Study the drawing (mm; zero at the part's minimum x, y, z) and answer. A direction names the side the tool comes from. Give positions to 0.01 mm unless a question says otherwise; leave off trailing zeros. Order: outer loops, then holes, each group sorted by start corner. A loop starts at its lowest first (then second) coordinate and runs counter-clockwise, first axis right, second up. Notation, with made-up numbers: (-1, -29.75) - (29, -29.75) arc R20 cw to (29, -18.75) - close; hole circle Ø4 at (-30.75, -38). An arc over 180 degrees is marked (long way). Write each question's results on one line, items separated by ' | '. Start each with the question number.
Q1. Find section A-A on z = 34.5. Count the separate pieces of the cut face and the enclosed holes in it, and give its area (3 significant figures).
Q2. Flat-ended cylindrical pins translate along their axes: P1, Ø1.5, axis at y = 34, z = 28, coming from the +X side; P2, Ø4, axis at x = 91.5, z = 8.5, coming from the -Y side. Find the tip coordinate at first contact, or state that the pin passes through.
Q3. Find section B-B on y = 6.5. Give the vertices of the cut face in (x, z).
Q4. Find section D-D on x = 118.5. Give the vertices of the cut face in (y, z), and give its area (3 significant figures).
Q5. Find section C-C on x = 6. Give the vertices of the cut face in (y, z), and give its area (3 significant figures).
Q6. A tool of negligible diameter and unlimited length cuts with its end or side. For the marked faces 1, 2 and 3, from which of +Z, -Z, +X, -X, +Y, -Y can it reach the whole face along a straight path? Write none if from no direction.
Q7. Find the intervals of material crossed by line 1 along X through (y, z) = (6, 23); line 2 along Y through (x, z) = (6, 41.5); line 3 along Y through (x, z) = (80.5, 32.5), in increasing order. Write a range as from..to.
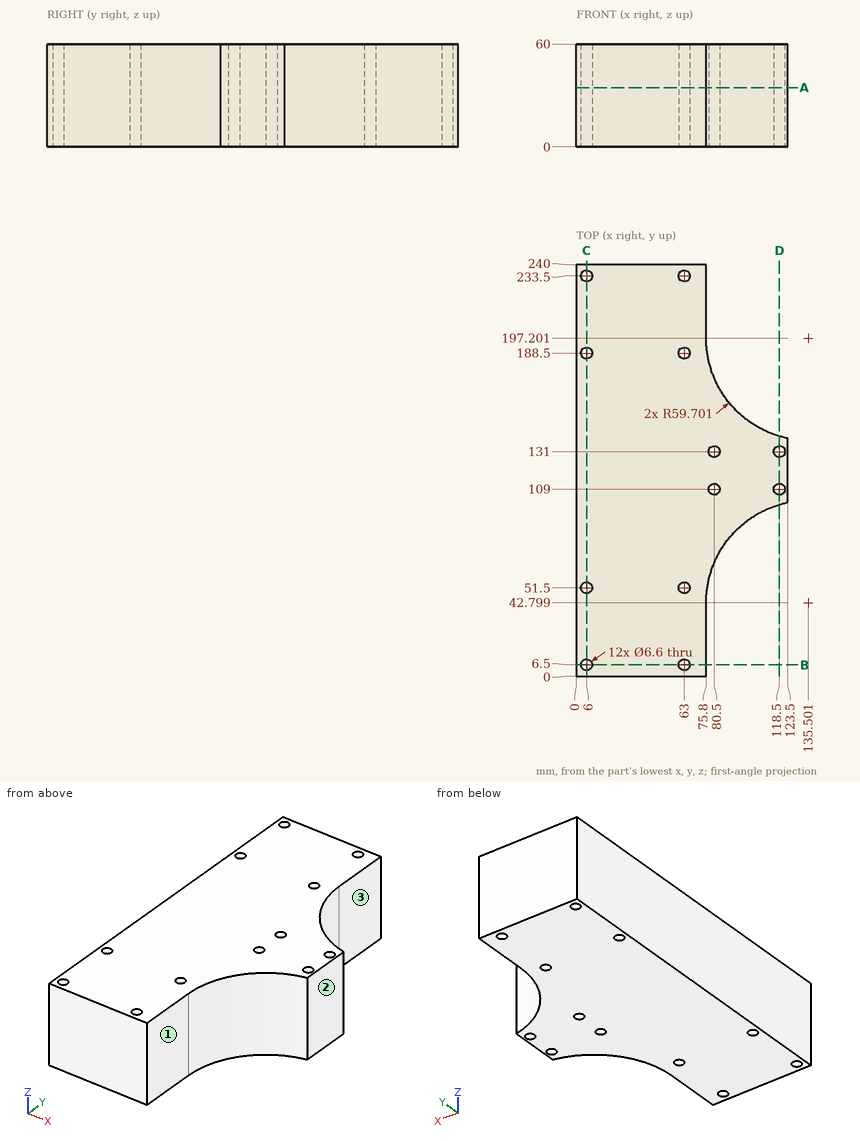
Working result:
1) separate pieces: 1 | enclosed holes: 12 | area: 21,000 mm²
2) P1: x = 75.8 | P2: y = 80.85
3) outline: (0, 0) - (2.7, 0) - (2.7, 60) - (0, 60) - close; (9.3, 0) - (59.7, 0) - (59.7, 60) - (9.3, 60) - close; (66.3, 0) - (75.8, 0) - (75.8, 60) - (66.3, 60) - close
4) outline: (100.03, 0) - (105.7, 0) - (105.7, 60) - (100.03, 60) - close; (112.3, 0) - (127.7, 0) - (127.7, 60) - (112.3, 60) - close; (134.3, 0) - (139.97, 0) - (139.97, 60) - (134.3, 60) - close | area: 1,600 mm²
5) outline: (0, 0) - (3.2, 0) - (3.2, 60) - (0, 60) - close; (9.8, 0) - (48.2, 0) - (48.2, 60) - (9.8, 60) - close; (54.8, 0) - (185.2, 0) - (185.2, 60) - (54.8, 60) - close; (191.8, 0) - (230.2, 0) - (230.2, 60) - (191.8, 60) - close; (236.8, 0) - (240, 0) - (240, 60) - (236.8, 60) - close | area: 12,800 mm²
6) face 1: +Z, -Z, +X, -Y | face 2: +Z, -Z, +X, +Y, -Y | face 3: +Z, -Z, +X, +Y
7) line 1: 0..2.74, 9.26..59.74, 66.26..75.8 | line 2: 0..3.2, 9.8..48.2, 54.8..185.2, 191.8..230.2, 236.8..240 | line 3: 66.02..105.7, 112.3..127.7, 134.3..173.98
